Geometry check sheet. Reference: the model listing, model coordinates, mm. Face numbers are marked on the shaded views. Give positions to 0.01 mm unless a question says otherwise; leave off trailing zeros. Order: outer loops, then holes, each group sorted by start corner. A loop starts at its lowest first (then second) coordinate and runs counter-clockwise, first axis right, second up. Notation, with made-up numbers: M -36.5,69.25 L -17.5,69.25 A21 ccw -17.5,82.25 Z; hole C 42,8.25 d9. An arc over 180 degrees is marked long. Put each result on its own line as item: value. Start each with the question number.
Q1. Material ranges on L1, parallel to Y at x = 0, z = 63; L2, parallel to Y at x = -22, z = 51.5; L3, parallel to Z at x = -11.5, y = 18.5, recorded low to high.
Q2. Mould release check, pull along X, two halves, no side actions. Record for the marked faces 1, 2 and 3: +X half, -X half, draft (parallel to the pull), parting line (faces both ways), or undercut.
Q3. Section check A-A on z = 41. Record the cut outline in (x, y), then the cut area to 3 significant figures.
Q4. Go/stop test with flat-tipped pins: pin 1 (2 mm diameter, centred on x = 11, y = 19.5, fed in from -Z); pin 2 (10 mm diameter, centred on y = 7.5, z = 29, fed in from -X); pin 3 (1.5 mm diameter, centred on x = 18.5, y = 5, fed in from +Z). Record where each tip stops, or that it passes through.
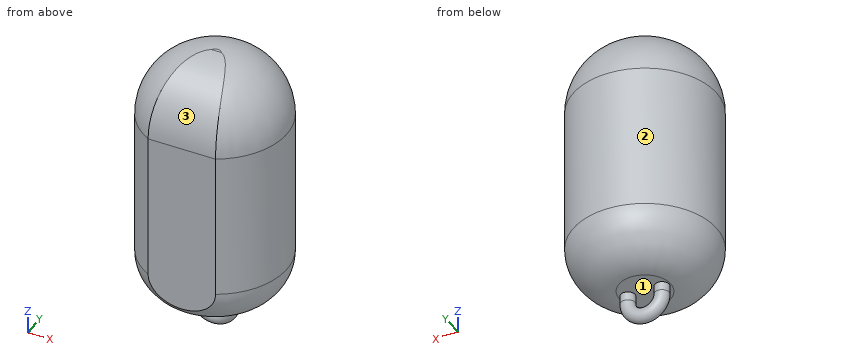
```python
from build123d import *

# Parameters (mm, degrees)
CROQUIS1_R              = 25
SALIENTE_EXTRUIR1_DEPTH = 90
CROQUIS4_R              = 2.5
REDONDEO2_R             = 16
CORTAR_EXTRUIR2_START   = -22
CROQUIS12_W             = 90
CROQUIS12_H             = 90
CORTAR_EXTRUIR2_DEPTH   = 30
REDONDEO3_R             = 23


with BuildPart() as part:
    # Croquis1 → Saliente-Extruir1 (new body)
    with BuildSketch(Plane.XY):
        with Locations(Location((0, 0, 0), (0, 0, 180))):
            Circle(CROQUIS1_R)
    extrude(amount=SALIENTE_EXTRUIR1_DEPTH)

    # Barrer3: sweep along a path in Croquis3
    with BuildLine(Plane(origin=(0, 0, 0), x_dir=(1, 0, 0), z_dir=(0, 1, 0))) as barrer3_path:
        Line((-3, 0), (-3, 3))
        ThreePointArc((-3, 3), (0, 6), (3, 3))
        Line((3, 3), (3, 0))
    # Croquis4 → Barrer3 (sweep)
    with BuildSketch(Plane(origin=(0, 0, 0), x_dir=(-1, 0, 0), z_dir=(0, 0, -1))):
        with Locations((-6, 0)):
            Circle(CROQUIS4_R)
    sweep(path=barrer3_path.line)

    # Redondeo2
    redondeo2_edges = [part.edges().sort_by_distance(p)[0] for p in [
        (25, 0, 0),
    ]]
    fillet(redondeo2_edges, radius=REDONDEO2_R)

    # Croquis12 → Cortar-Extruir2 (cut)
    with BuildSketch(Plane(origin=(0, 0, 0), x_dir=(1, 0, 0), z_dir=(0, 1, 0)).offset(CORTAR_EXTRUIR2_START)):
        with Locations((-20, -45)):
            Rectangle(CROQUIS12_W, CROQUIS12_H)
    extrude(amount=-CORTAR_EXTRUIR2_DEPTH, mode=Mode.SUBTRACT)

    # Redondeo3
    # the kernel refuses this fillet: 23 mm, written as the material it takes off along each edge
    with BuildSketch(Plane(origin=(0, 0, 90), x_dir=(-0.003141587485819883, -0.9999950652018583, 0), z_dir=(0.9999950652018583, -0.003141587485819883, 0))) as redondeo3_piece_1:
        with BuildLine():
            CenterArc((25 - REDONDEO3_R, REDONDEO3_R), REDONDEO3_R, 270, 90)
            Line((25 - REDONDEO3_R, 0), (25, 0))
            Line((25, 0), (25, REDONDEO3_R))
        make_face()
    revolve(axis=Axis((0, 0, 90), (0, 0, -1)), revolution_arc=359.64, mode=Mode.SUBTRACT)
    with BuildSketch(Plane(origin=(69.374342087, -22, 90), x_dir=(0, 1, 0), z_dir=(-1, 0, 0))) as redondeo3_piece_2:
        with BuildLine():
            CenterArc((REDONDEO3_R, REDONDEO3_R), REDONDEO3_R, 180, 90)
            Line((0, REDONDEO3_R), (0, 0))
            Line((0, 0), (REDONDEO3_R, 0))
        make_face()
    extrude(amount=138.748684174, mode=Mode.SUBTRACT)


solid = part.part
```
Results found:
1. L1: y = -22 to 25
1. L2: y = -11.87 to 11.87
1. L3: z = 6.38 to 78.73
2. face 1: undercut
2. face 2: parting line
2. face 3: draft
3. outline: M -11.87,-22 L 11.87,-22 A25 ccw long Z
3. area: 1,920 mm^2
4. pin 1: stops at z = 5.87
4. pin 2: stops at x = -24.87
4. pin 3: stops at z = 83.11
